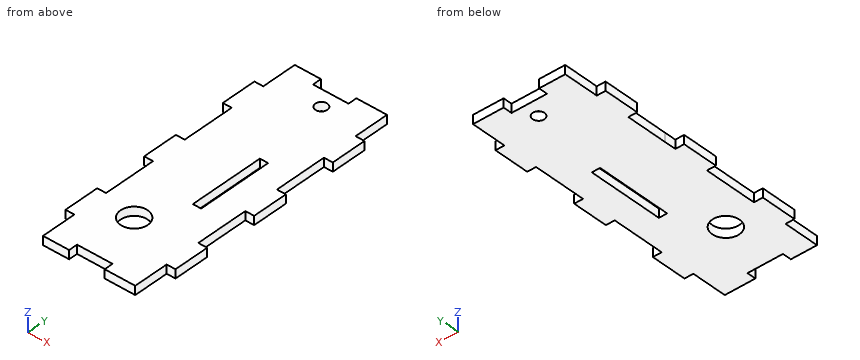
Autodesk Inventor part; units mm, degrees
ref_plane "YZ Plane" through (0, 0, 0) normal (1, 0, 0) x (0, 1, 0)
ref_plane "XZ Plane" through (0, 0, 0) normal (0, 1, 0) x (-1, 0, 0)
ref_plane "XY Plane" through (0, 0, 0) normal (0, 0, 1) x (1, 0, 0)
sketch "Boceto1" plane through (0, 0, 0) normal (0, 0, 1) x (-1, 0, 0)
  line L0 (-18.892, -36.3978) -> (-15.842, -36.3978)
  line L1 (-15.842, -36.3978) -> (-15.842, -48.4963)
  line L2 (-15.842, -48.4963) -> (-5.3194, -48.4963)
  line L3 (-5.3194, -48.4963) -> (-5.3194, -45.4463)
  line L4 (-5.3194, -45.4463) -> (6.8808, -45.4463)
  line L5 (6.8808, -45.4463) -> (6.8808, -48.4963)
  line L6 (6.8808, -48.4963) -> (9.213, -48.4963)
  line L7 (9.213, -48.4963) -> (15.8784, -48.4963)
  line L8 (15.8784, -48.4963) -> (15.8784, -47.9533)
  line L9 (15.8784, -47.9533) -> (15.8784, -45.4463)
  line L10 (15.8784, -45.4463) -> (15.8784, -36.3641)
  line L11 (15.8784, -36.3641) -> (18.9284, -36.3641)
  line L12 (18.9284, -36.3641) -> (18.9284, -24.1977)
  line L13 (18.9288, -24.1977) -> (15.8806, -24.1977)
  line L14 (15.8761, -24.2652) -> (15.8784, -24.1977)
  line L15 (15.8806, -24.1977) -> (15.8797, -10.139)
  line L16 (15.8797, -10.139) -> (15.8784, -6.1009)
  line L17 (15.8761, -6.1684) -> (15.8784, -6.1009)
  line L18 (15.8784, -6.1009) -> (18.9284, -6.1009)
  line L19 (18.9284, -6.1009) -> (18.9284, 6.0992)
  line L20 (18.9284, 6.0992) -> (15.8784, 6.0992)
  line L21 (15.8784, 6.0992) -> (15.8784, 24.1961)
  line L22 (15.8784, 24.1961) -> (18.9284, 24.1961)
  line L23 (18.9284, 24.1961) -> (18.9284, 36.3962)
  line L24 (18.9284, 36.3962) -> (15.8784, 36.3962)
  line L25 (15.8784, 36.3962) -> (15.8784, 45.4446)
  line L26 (15.8784, 45.4446) -> (15.8784, 48.4947)
  line L27 (15.8784, 48.4947) -> (6.8808, 48.4947)
  line L28 (6.8808, 48.4947) -> (6.8808, 45.4446)
  line L29 (6.8808, 45.4446) -> (-3.6418, 45.4446)
  line L30 (-3.6418, 45.4446) -> (-5.3194, 45.4446)
  line L31 (-5.3194, 45.4446) -> (-5.3194, 48.4947)
  line L32 (-5.3194, 48.4947) -> (-15.842, 48.4947)
  line L33 (-15.842, 48.4947) -> (-15.842, 36.3962)
  line L34 (-15.842, 36.3962) -> (-18.892, 36.3962)
  line L35 (-18.892, 36.3962) -> (-18.892, 24.1961)
  line L36 (-18.892, 24.1961) -> (-15.842, 24.1961)
  line L37 (-15.842, 24.1961) -> (-15.842, 6.0992)
  line L38 (-15.842, 6.0992) -> (-18.892, 6.0992)
  line L39 (-18.892, 6.0992) -> (-18.892, -6.1009)
  line L40 (-18.892, -6.1009) -> (-15.842, -6.1009)
  line L41 (-15.842, -6.1009) -> (-15.842, -24.1977)
  line L42 (-15.842, -24.1977) -> (-17.8753, -24.1977)
  line L43 (-17.8753, -24.1977) -> (-18.892, -24.1977)
  line L44 (-18.892, -24.1977) -> (-18.892, -36.3978)
  line L45 (-6.6919, -12.9634) -> (-6.6919, 12.8601)
  line L46 (-6.6919, 12.8601) -> (-3.8452, 12.8601)
  line L47 (-3.8452, 12.8601) -> (-3.8452, -12.9634)
  line L48 (-3.8452, -12.9634) -> (-6.6919, -12.9634)
  circle A0 centre (3.5759, 27.1591) radius 4.6767
  circle A1 centre (-0.9985, -39.8545) radius 2.0334
  point P0 (0, 0)
  dimension "d2" = 37.8204
  dimension "d3" = 96.991
extrude "Extrusión1" add sketch "Boceto1" along normal blind 3
properties part number "costat1"
Model file for the job. Use its own axes, mm. Give positions to 0.01 mm unless a question says otherwise; leave off trailing zeros. Write each loop counter-clockwise with the first axis right and the second up, starting at its lowest first coordinate (ties: lowest second). Pieces come first, ordered by that corner, then holes. Notation, with made-up numbers: (-3, 70.5) - (30, 70.5) arc R12 cw to (30, 84.5) - close; hole circle Ø7 at (68, -23). An arc over 180 degrees is marked (long way). One line per question, with ' | ' between items. Start each with the question number.
(1) Slice it at A-A on y = -11. Write the cut outline in (x, z), plus the area to 3 significant figures.
(2) Pin check, flat tips, straight feed: P1, Ø1.5, axis at y = -41.5, z = 1.5, coming from the -X side; P2, Ø0.9, axis at y = 45.5, z = 1.5, coming from the +X side; P3, Ø5.5, axis at x = -3.58, y = -27.16, coming from the -Z side; P4, Ø1.5, axis at x = -17, z = 1.5, coming from the +Y side. Stop position of each tip, or through.
(3) Slice it at B-B on x = -6. Write the cut outline in (y, z).
(4) Wall check: line 1 along Y through (x, z) = (16.5, 0.3); line 2 along X through (y, z) = (-2, 1.45); line 3 along X through (y, z) = (-7.5, 1.75). Give the ranges that are in metal, low to high. Write a range as from..to.
(5) Slice it at C-C on z = 2.25. Give the number of separate pieces and of enclosed holes in the cut face, plus the area to 3 significant figures.
Results below:
1) outline: (-15.88, 0) - (3.85, 0) - (3.85, 3) - (-15.88, 3) - close; (6.69, 0) - (15.84, 0) - (15.84, 3) - (6.69, 3) - close | area: 86.6 mm^2
2) P1: x = -15.88 | P2: x = 15.84 | P3: through | P4: y = 36.36
3) outline: (-45.44, 0) - (-31.16, 0) - (-31.16, 3) - (-45.44, 3) - close; (-23.16, 0) - (45.45, 0) - (45.45, 3) - (-23.16, 3) - close
4) line 1: -36.4..-24.2, -6.1..6.1, 24.2..36.4 | line 2: -18.93..3.85, 6.69..18.89 | line 3: -15.88..3.85, 6.69..15.84
5) separate pieces: 1 | enclosed holes: 3 | area: 3,070 mm^2
